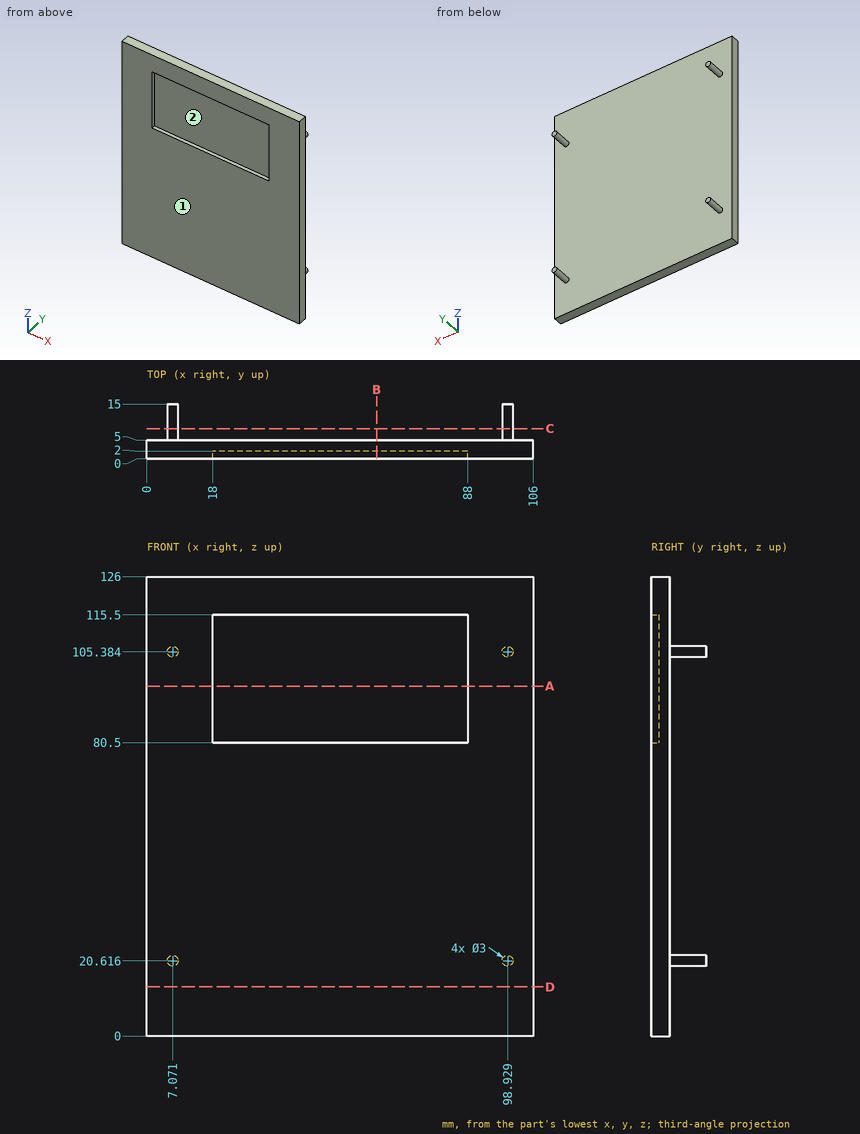
Here's the drawing with two shaded views (mm, measured from the low corner). I have some questions. Give positions to 0.01 mm unless a question says otherwise; leave off trailing zeros. Loops run counter-clockwise (first coordinate to the right, second up) from the corner with the lowest first, then second, coordinate; pieces in that order, holes last. Notation, with made-up numbers: (49, -37.75) - (85, -37.75) arc R31 ccw to (85, -11.75) - close; hole circle Ø11 at (57.25, 23.5). An arc over 180 degrees is marked (long way). Return JSON: item names as keys, results as strings.
1. We'd pull the mould along Z, two halves only. Please class the marked faces 1 and 2: +Z half, -Z half, draft (parallel to the pull), parting line (faces both ways), or undercut.
Output values:
{"face 1": "draft", "face 2": "undercut"}
2. If I drill on line 1 (X direction, y = 1.5, z = 109); line 2 (Y direction, x = 63, z = 55); line 3 (Y direction, x = 59, z = 86.5), over which ranges is the centre line in solid material (lowest first)?
Output values:
{"line 1": "x = 0 to 18, 88 to 106", "line 2": "y = 0 to 5", "line 3": "y = 2 to 5"}
3. I want a section at D-D on z = 13.5. Please give me the cut outline in (x, y), and give its area (3 significant figures).
Output values:
{"outline": "(0, 0) - (106, 0) - (106, 5) - (0, 5) - close", "area": "530 mm²"}
4. I'm going to push flat-ended pins straight in: pin 1 Ø1.6 at (x, y) = (49.5, 1) entering from -Z; pin 2 Ø17.5 at (x, z) = (69, 106.5) entering from -Y; pin 3 Ø4 at (y, z) = (8.5, 88.5) entering from +X; pin 4 Ø1 at (x, z) = (38.5, 57) entering from +Y. Where does each tip first touch, or does it pass through?
Output values:
{"pin 1": "stops at z = 0", "pin 2": "stops at y = 2", "pin 3": "passes through", "pin 4": "stops at y = 5"}
5. I want a section at C-C on y = 8.25. Please give me the cut outline in (x, z).
Output values:
{"outline": "circle Ø3 at (7.07, 20.62); circle Ø3 at (7.07, 105.38); circle Ø3 at (98.93, 20.62); circle Ø3 at (98.93, 105.38)"}
6. I want a section at B-B on x = 63. Please give me the cut outline in (y, z).
Output values:
{"outline": "(0, 0) - (5, 0) - (5, 126) - (0, 126) - (0, 115.5) - (2, 115.5) - (2, 80.5) - (0, 80.5) - close"}
7. I want a section at A-A on z = 96. Please give me the cut outline in (x, y), and give its area (3 significant figures).
Output values:
{"outline": "(0, 0) - (18, 0) - (18, 2) - (88, 2) - (88, 0) - (106, 0) - (106, 5) - (0, 5) - close", "area": "390 mm²"}
